from build123d import *

# Parameters (mm, degrees)
BOSS_EXTRUDE1_DEPTH = 7.62
CUT_EXTRUDE4_DEPTH  = 65.443482206
SKETCH8_R           = 2.032
CUT_EXTRUDE6_DEPTH  = 65.443482206
SKETCH9_R           = 2.032
CUT_EXTRUDE7_DEPTH  = 25.4
SKETCH11_R          = 3.937
CUT_EXTRUDE9_DEPTH  = 2.286
SKETCH12_W          = 1.5875
SKETCH12_H          = 3.175
BOSS_EXTRUDE2_DEPTH = 7.62


with BuildPart() as part:
    # Sketch2 → Boss-Extrude1 (new body)
    with BuildSketch(Plane.XY):
        with BuildLine():
            Line((-53.9331315, -0.315391151), (-41.673792668, 33.030010472))
            ThreePointArc((-41.673792668, 33.030010472), (-41.022456018, 33.874587748), (-40.005, 34.194483756))
            Line((-40.005, 34.194483756), (40.005, 34.194483756))
            ThreePointArc((40.005, 34.194483756), (41.022456018, 33.874587748), (41.673792668, 33.030010472))
            Line((41.673792668, 33.030010472), (53.9331315, -0.315391151))
            ThreePointArc((53.9331315, -0.315391151), (54.072783991, -1.479661595), (53.674573059, -2.582592481))
            Line((53.674573059, -2.582592481), (39.780650937, -23.816388011))
            ThreePointArc((39.780650937, -23.816388011), (35.127277075, -28.095614939), (28.998611748, -29.64646397))
            Line((28.998611748, -29.64646397), (-28.998611748, -29.64646397))
            ThreePointArc((-28.998611748, -29.64646397), (-35.127277075, -28.095614939), (-39.780650937, -23.816388011))
            Line((-39.780650937, -23.816388011), (-53.674573059, -2.582592481))
            ThreePointArc((-53.674573059, -2.582592481), (-54.072783991, -1.479661595), (-53.9331315, -0.315391151))
        make_face()
    extrude(amount=BOSS_EXTRUDE1_DEPTH)

    # Sketch6 → Cut-Extrude4 (cut, through all)
    with BuildSketch(Plane.XY.offset(7.62)):
        with BuildLine():
            Line((-43.288518763, -7.189330581), (-32.273407011, -24.02349941))
            ThreePointArc((-32.273407011, -24.02349941), (-30.897448537, -25.288826187), (-29.085260384, -25.747397522))
            Line((-29.085260384, -25.747397522), (-16.452977044, -25.747397522))
            ThreePointArc((-16.452977044, -25.747397522), (-15.554951432, -25.375423134), (-15.182977044, -24.477397522))
            Line((-15.182977044, -24.477397522), (-15.182977044, -7.476646933))
            ThreePointArc((-15.182977044, -7.476646933), (-15.554951432, -6.578621321), (-16.452977044, -6.206646933))
            Line((-16.452977044, -6.206646933), (-42.757160992, -6.206646933))
            ThreePointArc((-42.757160992, -6.206646933), (-43.315732436, -6.539615574), (-43.288518763, -7.189330581))
        make_face()
        with BuildLine():
            Line((43.288518763, -7.189330581), (32.273407011, -24.02349941))
            ThreePointArc((32.273407011, -24.02349941), (30.897448537, -25.288826187), (29.085260384, -25.747397522))
            Line((29.085260384, -25.747397522), (16.452977044, -25.747397522))
            ThreePointArc((16.452977044, -25.747397522), (15.554951432, -25.375423134), (15.182977044, -24.477397522))
            Line((15.182977044, -24.477397522), (15.182977044, -7.476646933))
            ThreePointArc((15.182977044, -7.476646933), (15.554951432, -6.578621321), (16.452977044, -6.206646933))
            Line((16.452977044, -6.206646933), (42.757160992, -6.206646933))
            ThreePointArc((42.757160992, -6.206646933), (43.315732436, -6.539615574), (43.288518763, -7.189330581))
        make_face()
    extrude(amount=-CUT_EXTRUDE4_DEPTH, mode=Mode.SUBTRACT)

    # Sketch8 → Cut-Extrude6 (cut, through all)
    with BuildSketch(Plane.XY.offset(7.62)):
        with Locations((-40.64, 3.445353067)):
            Circle(SKETCH8_R)
        with Locations((-34.29, 24.273353067)):
            Circle(SKETCH8_R)
        with Locations((40.64, 3.445353067)):
            Circle(SKETCH8_R)
        with Locations((34.29, 24.273353067)):
            Circle(SKETCH8_R)
    extrude(amount=-CUT_EXTRUDE6_DEPTH, mode=Mode.SUBTRACT)

    # Sketch9 → Cut-Extrude7 (cut)
    with BuildSketch(Plane.XZ.offset(29.64646397)):
        with Locations(Location((0, 3.81, 0), (0, 0, 270))):
            Circle(SKETCH9_R)
    extrude(amount=-CUT_EXTRUDE7_DEPTH, mode=Mode.SUBTRACT)

    # Sketch11 → Cut-Extrude9 (cut)
    with BuildSketch(Plane.XY.offset(7.62)):
        with Locations((-34.29, 24.273353067)):
            Circle(SKETCH11_R)
        with Locations((-40.64, 3.445353067)):
            Circle(SKETCH11_R)
        with Locations(Location((40.64, 3.445353067, 0), (0, 0, 180))):
            Circle(SKETCH11_R)
        with Locations(Location((34.29, 24.273353067, 0), (0, 0, 180))):
            Circle(SKETCH11_R)
    extrude(amount=-CUT_EXTRUDE9_DEPTH, mode=Mode.SUBTRACT)

    # Sketch12 → Boss-Extrude2 (add)
    with BuildSketch(Plane.XY.offset(7.62)):
        with Locations((-4.7625, -31.23396397)):
            Rectangle(SKETCH12_W, SKETCH12_H)
        with Locations((4.7625, -31.23396397)):
            Rectangle(SKETCH12_W, SKETCH12_H)
    extrude(amount=-BOSS_EXTRUDE2_DEPTH)


solid = part.part
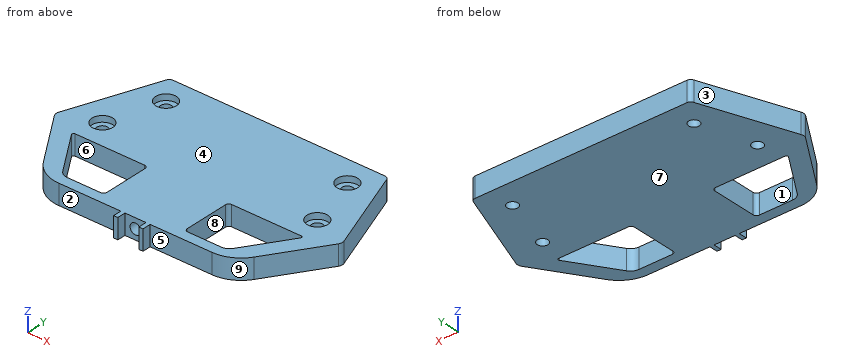
Could you check a few things on this model? Use its own coordinates, in mm. Face numbers are marked on the shaded views. A direction names the side the tool comes from. Give positions to 0.01 mm unless a question says otherwise; leave off trailing zeros. Order: outer loops, then holes, each group sorted by start corner. A loop starts at its lowest first (then second) coordinate and runs counter-clockwise, first axis right, second up. Notation, with made-up numbers: (42.5, 87) - (72.5, 87) arc R26 ccw to (72.5, 105) - close; hole circle Ø3 at (3, -13). An arc over 180 degrees is marked (long way). Return JSON: item names as keys, results as strings. Group by question number.
Q1. Which directions (+Z, -Z, +X, -X, +Y, -Y) give clear straight access to the entire face, cutting with the end or side of a thin tool? Please do the marked faces 1, 2, 3, 4 and 5.
Q2. Suppose I cut it at A-A, the plane y = -21.5. Please give me the cut outline in (x, z).
Q3. Suppose I cut it at B-B, the plane x = 23.5. Please give me the cut outline in (y, z), and give its area (3 significant figures).
Q4. Suppose I cut it at D-D, the plane x = 0. Please give me the cut outline in (y, z).
Q5. Thinking about a two-plate mould opening in Y: for the marked faces 6, 7, 8 and 9, which applies, pulls with the +Y half, pulls with the -Y half, needs draft (parallel to the pull), parting line crosses it, or undercut?
Q6. Will these pins go through, and if not, where does the flat tip stop? pin 1 Ø1.6 at (y, z) = (-31.5, 5.5) entering from -X; pin 2 Ø2.5 at (x, z) = (0, 3.81) entering from -Y; pin 3 Ø1 at (y, z) = (-30.5, 4) entering from +X.
Q7. Suppose I cut it at C-C, the plane x = -34.29. Please give me the cut outline in (y, z), and give its area (3 significant figures).
Q8. Please list where these lines run through material, in increasing order: line 1 along Y through (x, z) = (-36, 2); line 2 along Y through (x, z) = (-34.29, 7); line 3 along X through (y, z) = (1.5, 5.75). Write a range as [from, to].
Resolved:
{
 "1": {"face 1": "+Z, -Z", "face 2": "+Z, -Z, -X, -Y", "face 3": "+Z, -Z, -X, +Y", "face 4": "+Z, +X, -X, +Y, -Y", "face 5": "+Z, -Z, +X, -Y"},
 "2": {"outline": "(-41.3, 0) - (-33.92, 0) - (-33.92, 7.62) - (-41.3, 7.62) - close; (-15.18, 0) - (15.18, 0) - (15.18, 7.62) - (-15.18, 7.62) - close; (33.92, 0) - (41.3, 0) - (41.3, 7.62) - (33.92, 7.62) - close; hole circle Ø4.06 at (0, 3.81)"},
 "3": {"outline": "(-29.65, 0) - (-25.75, 0) - (-25.75, 7.62) - (-29.65, 7.62) - close; (-6.21, 0) - (34.19, 0) - (34.19, 7.62) - (-6.21, 7.62) - close", "area": "338 mm2"},
 "4": {"outline": "(-29.65, 0) - (34.19, 0) - (34.19, 7.62) - (-29.65, 7.62) - (-29.65, 5.84) - (-4.25, 5.84) - (-4.25, 1.78) - (-29.65, 1.78) - close"},
 "5": {"face 6": "undercut", "face 7": "needs draft", "face 8": "undercut", "face 9": "pulls with the -Y half"},
 "6": {"pin 1": "stops at x = -5.56", "pin 2": "stops at y = -4.25", "pin 3": "stops at x = 5.56"},
 "7": {"outline": "(-28.51, 0) - (-20.94, 0) - (-20.94, 7.62) - (-28.51, 7.62) - close; (-6.21, 0) - (22.24, 0) - (22.24, 5.33) - (20.34, 5.33) - (20.34, 7.62) - (-6.21, 7.62) - close; (26.31, 0) - (34.19, 0) - (34.19, 7.62) - (28.21, 7.62) - (28.21, 5.33) - (26.31, 5.33) - close", "area": "326 mm2"},
 "8": {"line 1": "y = [-27.58, -18.33], [-6.21, 23.18], [25.37, 34.19]", "line 2": "y = [-28.51, -20.94], [-6.21, 20.34], [28.21, 34.19]", "line 3": "x = [-53.27, -44.06], [-37.22, 37.22], [44.06, 53.27]"}
}
